from build123d import *

# Parameters (mm, degrees)
EXTRUDE_1_DEPTH      = 6
SKETCH_2_R           = 16
CUT_EXTRUDE_1_DEPTH  = 5
CHAMFER_1_SIZE       = 0.5
CHAMFER_1_SIZE2      = 1.025151921
SKETCH_24_R          = 15
CUT_EXTRUDE_15_DEPTH = 149.618639477
CUT_EXTRUDE_16_DEPTH = 4
SKETCH_26_W          = 1
SKETCH_26_H          = 8
CUT_EXTRUDE_17_DEPTH = 149.655642342
SKETCH_27_R          = 1.35
CUT_EXTRUDE_18_DEPTH = 152.486798105
SKETCH_29_W          = 33
SKETCH_29_H          = 6
EXTRUDE_3_DEPTH      = 12
EXTRUDE_4_DEPTH      = 2
EXTRUDE_5_DEPTH      = 9
SKETCH_32_W          = 24.73
SKETCH_32_H          = 50
CUT_EXTRUDE_19_DEPTH = 4
SKETCH_33_W          = 14.3
SKETCH_33_H          = 2.35
CUT_EXTRUDE_20_DEPTH = 1.5
EXTRUDE_6_REACH      = 119.22
SKETCH_34_W          = 5.215
SKETCH_34_H          = 3
CUT_EXTRUDE_START    = -6
CUT_EXTRUDE_21_DEPTH = 6
SKETCH_36_R          = 1.15
CUT_EXTRUDE_22_DEPTH = 150.192828246
SKETCH_37_R          = 16
CUT_EXTRUDE_23_DEPTH = 5
SKETCH_38_R          = 15
CUT_EXTRUDE_24_DEPTH = 150.504180544
CUT_EXTRUDE_25_DEPTH = 4
SKETCH_40_W          = 33
SKETCH_40_H          = 10
EXTRUDE_7_DEPTH      = 22.1
SKETCH_41_W          = 15.2
SKETCH_41_H          = 3
CUT_EXTRUDE_26_DEPTH = 7.8
SKETCH_42_R          = 1.35
CUT_EXTRUDE_27_DEPTH = 8
SKETCH_43_W          = 6.5
SKETCH_43_H          = 3
EXTRUDE_8_DEPTH      = 29
CUT_EXTRUDE_28_REACH = 154.858
SKETCH_48_R          = 1.35
RIB_START            = -1.5
RIB_17_DEPTH         = 1.5
RIB_20_DEPTH         = 1.5
CHAMFER_2_SIZE       = 1


# Read off the part's stored shape, not the designer's step: 보강대17, 보강대20
with BuildPart() as part:
    # 스케치1 → 보스-돌출1 (new body)
    with BuildSketch(Plane.XY):
        with BuildLine():
            Line((-17.5, 0), (-17.5, 130))
            ThreePointArc((-17.5, 130), (0, 147.5), (17.5, 130))
            Line((17.5, 130), (17.5, 0))
            ThreePointArc((17.5, 0), (0, -17.5), (-17.5, 0))
        make_face()
    extrude(amount=EXTRUDE_1_DEPTH)

    # 스케치2 → 컷-돌출1 (cut)
    with BuildSketch(Plane(origin=(0, 0, 0), x_dir=(-1, 0, 0), z_dir=(0, 0, -1))):
        with Locations((0, 130)):
            Circle(SKETCH_2_R)
    extrude(amount=-CUT_EXTRUDE_1_DEPTH, mode=Mode.SUBTRACT)

    # 모따기1
    chamfer_1_edges = [part.edges().sort_by_distance(p)[0] for p in [
        (16, 130, 0),
    ]]
    chamfer_1_side = [part.faces().sort_by_distance(p)[0] for p in [
        (16, 130, 2.5),
    ]]
    chamfer(chamfer_1_edges, length=CHAMFER_1_SIZE, length2=CHAMFER_1_SIZE2, reference=chamfer_1_side[0])

    # 스케치24 → 컷-돌출15 (cut, through all)
    with BuildSketch(Plane(origin=(0, 0, 5), x_dir=(-1, 0, 0), z_dir=(0, 0, -1))):
        with Locations((0, 130)):
            Circle(SKETCH_24_R)
    extrude(amount=-CUT_EXTRUDE_15_DEPTH, mode=Mode.SUBTRACT)

    # 스케치25 → 컷-돌출16 (cut)
    with BuildSketch(Plane.XY.offset(6)):
        with BuildLine():
            Line((-15.5, 97), (15.5, 97))
            Line((15.5, 97), (15.5, 117.36077534))
            ThreePointArc((15.5, 117.36077534), (0, 110), (-15.5, 117.36077534))
            Line((-15.5, 117.36077534), (-15.5, 97))
        make_face()
        Polygon((-15.5, 79), (-12.5, 79), (-12.5, 91), (12.5, 91), (12.5, 79), (15.5, 79), (15.5, 68), (-15.5, 68), align=None)
    extrude(amount=-CUT_EXTRUDE_16_DEPTH, mode=Mode.SUBTRACT)

    # 스케치26 → 컷-돌출17 (cut, through all)
    with BuildSketch(Plane.XY.offset(6)):
        with Locations((-17, 87)):
            Rectangle(SKETCH_26_W, SKETCH_26_H)
        with Locations((17, 87)):
            Rectangle(SKETCH_26_W, SKETCH_26_H)
        with Locations((-17, 35)):
            Rectangle(SKETCH_26_W, SKETCH_26_H)
        with Locations((17, 35)):
            Rectangle(SKETCH_26_W, SKETCH_26_H)
    extrude(amount=-CUT_EXTRUDE_17_DEPTH, mode=Mode.SUBTRACT)

    # 스케치27 → 컷-돌출18 (cut, through all)
    with BuildSketch(Plane.ZY.offset(16.5)):
        with Locations((3.5, 87)):
            Circle(SKETCH_27_R)
        with Locations(Location((2.5, 35, 0), (0, 0, 270))):
            Circle(SKETCH_27_R)
    extrude(amount=-CUT_EXTRUDE_18_DEPTH, mode=Mode.SUBTRACT)

    # 스케치29 → 보스-돌출3 (add)
    with BuildSketch(Plane.XY.offset(6)):
        with Locations((0, 94)):
            Rectangle(SKETCH_29_W, SKETCH_29_H)
    extrude(amount=EXTRUDE_3_DEPTH)

    # 스케치30 → 보스-돌출4 (add)
    with BuildSketch(Plane.XY.offset(6)):
        with BuildLine():
            Line((-17.5, 130), (-15, 130))
            ThreePointArc((-15, 130), (0, 145), (15, 130))
            Line((15, 130), (17.5, 130))
            ThreePointArc((17.5, 130), (0, 147.5), (-17.5, 130))
        make_face()
    extrude(amount=EXTRUDE_4_DEPTH)

    # 스케치31 → 보스-돌출5 (add)
    with BuildSketch(Plane.XY.offset(8)):
        with BuildLine():
            Line((-17.5, 130), (-11, 130))
            ThreePointArc((-11, 130), (-9.257654472, 135.941029682), (-4.582575695, 140))
            Line((-4.582575695, 140), (-14.361406616, 140))
            ThreePointArc((-14.361406616, 140), (-16.696925103, 135.240485866), (-17.5, 130))
        make_face()
        with BuildLine():
            Line((11, 130), (17.5, 130))
            ThreePointArc((17.5, 130), (16.696925103, 135.240485866), (14.361406616, 140))
            Line((14.361406616, 140), (4.582575695, 140))
            ThreePointArc((4.582575695, 140), (9.257654472, 135.941029682), (11, 130))
        make_face()
    extrude(amount=EXTRUDE_5_DEPTH)

    # 스케치32 → 컷-돌출19 (cut)
    with BuildSketch(Plane.XY.offset(18)):
        with Locations((0, 119.65)):
            Rectangle(SKETCH_32_W, SKETCH_32_H)
    extrude(amount=-CUT_EXTRUDE_19_DEPTH, mode=Mode.SUBTRACT)

    # 스케치33 → 컷-돌출20 (cut)
    with BuildSketch(Plane.XY.offset(14)):
        with Locations((0, 95.825)):
            Rectangle(SKETCH_33_W, SKETCH_33_H)
    extrude(amount=-CUT_EXTRUDE_20_DEPTH, mode=Mode.SUBTRACT)

    # 스케치34 → 보스-돌출6 (add, up to next)
    with BuildSketch(Plane(origin=(0, 97, 0), x_dir=(1, 0, 0), z_dir=(0, 1, 0)), mode=Mode.PRIVATE) as extrude_6_sk1:
        with Locations((-9.7575, -12.5)):
            Rectangle(SKETCH_34_W, SKETCH_34_H)
    extrude_6_tool1 = extrude(extrude_6_sk1.sketch, amount=EXTRUDE_6_REACH, mode=Mode.PRIVATE) - part.part
    # 스케치34 → 보스-돌출6 (add, up to next)
    with BuildSketch(Plane(origin=(0, 97, 0), x_dir=(1, 0, 0), z_dir=(0, 1, 0)), mode=Mode.PRIVATE) as extrude_6_sk2:
        with Locations((9.7575, -12.5)):
            Rectangle(SKETCH_34_W, SKETCH_34_H)
    extrude_6_tool2 = extrude(extrude_6_sk2.sketch, amount=EXTRUDE_6_REACH, mode=Mode.PRIVATE) - part.part
    add(extrude_6_tool1.solids().sort_by_distance((-9.7575, 97, 12.5))[0])
    add(extrude_6_tool2.solids().sort_by_distance((9.7575, 97, 12.5))[0])

    # 스케치35 → 컷-돌출21 (cut)
    with BuildSketch(Plane.XY.offset(14).offset(CUT_EXTRUDE_START)):
        with BuildLine():
            Line((-11, 130), (-11, 140))
            Line((-11, 140), (11, 140))
            Line((11, 140), (11, 130))
            ThreePointArc((11, 130), (0, 119), (-11, 130))
        make_face()
    extrude(amount=CUT_EXTRUDE_21_DEPTH, mode=Mode.SUBTRACT)

    # 스케치36 → 컷-돌출22 (cut, through all)
    with BuildSketch(Plane.XY.offset(14)):
        with Locations((-10.25, 121.15)):
            Circle(SKETCH_36_R)
        with Locations((10.25, 121.15)):
            Circle(SKETCH_36_R)
        with Locations((-10.25, 100.65)):
            Circle(SKETCH_36_R)
        with Locations((10.25, 100.65)):
            Circle(SKETCH_36_R)
    extrude(amount=-CUT_EXTRUDE_22_DEPTH, mode=Mode.SUBTRACT)

    # 스케치37 → 컷-돌출23 (cut)
    with BuildSketch(Plane.XY.offset(6)):
        Circle(SKETCH_37_R)
    extrude(amount=-CUT_EXTRUDE_23_DEPTH, mode=Mode.SUBTRACT)

    # 스케치38 → 컷-돌출24 (cut, through all)
    with BuildSketch(Plane.XY.offset(1)):
        Circle(SKETCH_38_R)
    extrude(amount=-CUT_EXTRUDE_24_DEPTH, mode=Mode.SUBTRACT)

    # 스케치39 → 컷-돌출25 (cut)
    with BuildSketch(Plane(origin=(0, 0, 0), x_dir=(-1, 0, 0), z_dir=(0, 0, -1))):
        with BuildLine():
            Line((-15.5, 58), (-15.5, 41))
            Line((-15.5, 41), (-13.5, 41))
            Line((-13.5, 41), (-13.5, 29))
            Line((-13.5, 29), (-15.5, 29))
            Line((-15.5, 29), (-15.5, 12.63922466))
            ThreePointArc((-15.5, 12.63922466), (0, 20), (15.5, 12.63922466))
            Line((15.5, 12.63922466), (15.5, 29))
            Line((15.5, 29), (13.5, 29))
            Line((13.5, 29), (13.5, 41))
            Line((13.5, 41), (15.5, 41))
            Line((15.5, 41), (15.5, 58))
            Line((15.5, 58), (-15.5, 58))
        make_face()
    extrude(amount=-CUT_EXTRUDE_25_DEPTH, mode=Mode.SUBTRACT)

    # 스케치40 → 보스-돌출7 (add)
    with BuildSketch(Plane(origin=(0, 0, 4), x_dir=(-1, 0, 0), z_dir=(0, 0, -1))):
        with Locations((0, 26)):
            Rectangle(SKETCH_40_W, SKETCH_40_H)
    extrude(amount=EXTRUDE_7_DEPTH)

    # 스케치41 → 컷-돌출26 (cut)
    with BuildSketch(Plane(origin=(0, 0, -18.1), x_dir=(-1, 0, 0), z_dir=(0, 0, -1))):
        with Locations((0, 22.5)):
            Rectangle(SKETCH_41_W, SKETCH_41_H)
    extrude(amount=-CUT_EXTRUDE_26_DEPTH, mode=Mode.SUBTRACT)

    # 스케치42 → 컷-돌출27 (cut)
    with BuildSketch(Plane(origin=(0, 0, -18.1), x_dir=(-1, 0, 0), z_dir=(0, 0, -1))):
        with Locations((-3.75, 27.33)):
            Circle(SKETCH_42_R)
        with Locations((3.75, 27.33)):
            Circle(SKETCH_42_R)
    extrude(amount=-CUT_EXTRUDE_27_DEPTH, mode=Mode.SUBTRACT)

    # 스케치43 → 보스-돌출8 (add)
    with BuildSketch(Plane.XZ.offset(-21)):
        with Locations((-10.85, -16.6)):
            Rectangle(SKETCH_43_W, SKETCH_43_H)
        with Locations((10.85, -16.6)):
            Rectangle(SKETCH_43_W, SKETCH_43_H)
    extrude(amount=EXTRUDE_8_DEPTH)

    # 스케치48 → 컷-돌출28 (cut, up to next)
    with BuildSketch(Plane(origin=(0, 0, -18.1), x_dir=(-1, 0, 0), z_dir=(0, 0, -1)), mode=Mode.PRIVATE) as cut_extrude_28_sk1:
        with Locations((10.8, -3.8)):
            Circle(SKETCH_48_R)
    cut_extrude_28_tool1 = extrude(cut_extrude_28_sk1.sketch, amount=-CUT_EXTRUDE_28_REACH, mode=Mode.PRIVATE) & part.part
    # 스케치48 → 컷-돌출28 (cut, up to next)
    with BuildSketch(Plane(origin=(0, 0, -18.1), x_dir=(-1, 0, 0), z_dir=(0, 0, -1)), mode=Mode.PRIVATE) as cut_extrude_28_sk2:
        with Locations((-10.8, -3.8)):
            Circle(SKETCH_48_R)
    cut_extrude_28_tool2 = extrude(cut_extrude_28_sk2.sketch, amount=-CUT_EXTRUDE_28_REACH, mode=Mode.PRIVATE) & part.part
    add(cut_extrude_28_tool1.solids().sort_by_distance((-10.8, -3.8, -18.1))[0], mode=Mode.SUBTRACT)
    add(cut_extrude_28_tool2.solids().sort_by_distance((10.8, -3.8, -18.1))[0], mode=Mode.SUBTRACT)

    # 보강대17 outline → 보강대17 (add)
    with BuildSketch(Plane(origin=(-7.6, 0, 0), x_dir=(0, 0, -1), z_dir=(1, 0, 0)).offset(RIB_START)):
        Polygon((15.1, -8), (15.1, 22), (-6, 22), (-6, 19.000000001), (-4, 18.011504048), (-3.591955232, 17.809828747), (0, 16.034512143), (10.186206897, 11), align=None)
    extrude(amount=RIB_17_DEPTH)

    # 보강대20 outline → 보강대20 (add)
    with BuildSketch(Plane.ZY.offset(-7.6).offset(RIB_START)):
        Polygon((-15.1, -8), (-10.186206897, 11), (0, 16.034512143), (3.591955232, 17.809828747), (4, 18.011504048), (4, 22), (-15.1, 22), align=None)
    extrude(amount=RIB_20_DEPTH)

    # 모따기2
    chamfer_2_edges = [part.edges().sort_by_distance(p)[0] for p in [
        (-11.4, 100.65, 0),
        (9.1, 100.65, 0),
    ]]
    chamfer(chamfer_2_edges, length=CHAMFER_2_SIZE)


solid = part.part
The listing builds one solid part. Answer for the finished solid, in the listing's coordinates (mm). A direction names the side the tool comes from. Give positions to 0.01 mm unless a question says otherwise; leave off trailing zeros. Order: outer loops, then holes, each group sorted by start corner. A loop starts at its lowest first (then second) coordinate and runs counter-clockwise, first axis right, second up. Notation, with made-up numbers: (12, 86) - (23, 86) arc R10 ccw to (23, 91) - close; hole circle Ø8 at (18, 47.25). An arc over 180 degrees is marked (long way). Use one line per item in the form item = value.
1) Find section A-A on x = 0. Give the number of separate pieces and of enclosed holes in the cut face, and give its area (3 significant figures).
Verdict:
separate_pieces = 3
enclosed_holes = 0
area = 575 mm^2
2) Find section B-B on y = 52. Determine the outline of the cut face in (x, z).
Verdict:
outline = (-17.5, 0) - (-15.5, 0) - (-15.5, 4) - (15.5, 4) - (15.5, 0) - (17.5, 0) - (17.5, 6) - (-17.5, 6) - close
3) Consider probe 1 along X at (y, z) = (16.5, -3.5); probe 2 along X at (y, z) = (46, 2.5); probe 3 along Z at (x, y) = (15, 35). Determine where each line is inside the solid, lowest interval first. Write a range as [from, to].
Verdict:
probe_1 = [-9.1, -7.6], [7.6, 9.1]
probe_2 = [-17.5, -15.5], [15.5, 17.5]
probe_3 = [0, 1.15], [3.85, 6]
4) Each of these flat-tipped pins is pushed along its axis until it touches: pin 1 (2.5 mm diameter, centred on x = -1.5, y = 22.5, fed in from -Z); pin 2 (3.5 mm diameter, centred on y = 136, z = 15, fed in from +X); pin 3 (2 mm diameter, centred on x = 2, y = 112.5, fed in from +Z). Where does it stop, or does it pass through?
Verdict:
pin_1 = -10.3
pin_2 = 16.98
pin_3 = 6
5) The mould has two halves that part along Y. Classify faces 5 (the flat face through (12.5, 85, 4)), 6 (the flat face through (-8.36, 13.552, -5.022)), 7 (the flat face through (-17.5, 61, 3)): released by +Y, released by -Y, zero draft, split by the parting line, or undercut.
Verdict:
face_5 = undercut
face_6 = released by -Y
face_7 = zero draft
6) For faces 1 (the flat face through (11, 135, 11)), 2 (the cylindrical face through (-3.574, 28.669, -14.156)), 3 (the flat face through (0, 38, 6)), 4 (the flat face through (10, 112, 14)), determine the directions among +Z, -Z, +X, -X, +Y, -Y from which every point of the face is accessible in a straight line to the end or side of a thin tool.
Verdict:
face_1 = +Z, -Z, +Y
face_2 = -Z
face_3 = +Z, +X, -X, -Y
face_4 = +Z, +Y
7) Find section C-C on z = -2.5. Determine the outline of the cut face in (x, y), and give its area (3 significant figures).
Verdict:
outline = (-16.5, 21) - (-9.1, 21) - (-9.1, 14.8) - (-7.6, 14.8) - (-7.6, 21) - (7.6, 21) - (7.6, 14.8) - (9.1, 14.8) - (9.1, 21) - (16.5, 21) - (16.5, 31) - (-16.5, 31) - close
area = 349 mm^2
